Part model, mm, in its own coordinate system. Give positions to 0.01 mm unless a question says otherwise; leave off trailing zeros. Write each loop counter-clockwise with the first axis right and the second up, starting at its lowest first coordinate (ties: lowest second). Pieces come first, ordered by that corner, then holes. Notation, with made-up numbers: M -25.75,9.25 L 32.25,9.25 A34 ccw 32.25,39.25 Z; hole C 22,28.25 d4. An arc over 180 degrees is marked long. Use CSV: the item, a comma, the result in double quotes. Start each with the question number.
Item 1: Mould opens along Y. For faces 1 (the flat face through (-14, 704.486, 30)), 2 (the cylindrical face through (7.331, 691.927, 29.671)), 3 (the flat face through (14.873, 689, 30)) say: released by +Y, released by -Y, zero draft, split by the parting line, or undercut.
Item 2: Drill centre lines: line 1 (X direction, y = 692.5, z = 19); line 2 (X direction, y = 691, z = -9); line 3 (Z direction, x = -22, y = 693). Where is each one in solid material? Low to high. Write a range as [from, to].
Item 3: Cut at A-A (x = -9). List the corners of the cut face in (y, z).
Item 4: Cut at D-D (z = 54.5). List the corners of the cut face in (x, y), then the cut area to 3 significant figures.
Item 5: Cut at B-B (z = 17). List the corners of the cut face in (x, y), then the cut area to 3 significant figures.
Item 6: Cut at C-C (y = 691). List the corners of the cut face in (x, z), then the cut area to 3 significant figures.
from build123d import *

# Parameters (mm, degrees)
BOSS_EXTRUDE1_DEPTH = 90
SKETCH3_R           = 11
CUT_EXTRUDE1_DEPTH  = 92.815774412
M6_TAPPED_HOLE_D    = 5


with BuildPart() as part:
    # Sketch1 → Boss-Extrude1 (new body)
    with BuildSketch(Plane(origin=(0, 2.518676762, -14.699029015), x_dir=(1, 0, 0), z_dir=(0, 0, 1))):
        Polygon((-43.126560257, 671.967635092), (-14.126560257, 671.967635092), (14.873439743, 671.967635092), (14.873439743, 701.967635092), (-43.126560257, 701.967635092), align=None)
    extrude(amount=BOSS_EXTRUDE1_DEPTH)

    # Sketch3 → Cut-Extrude1 (cut, through all)
    with BuildSketch(Plane.XZ.offset(-674.486311854)):
        with Locations(Location((-14.126560257, 15.300970985, 0), (0, 0, 270))):
            Circle(SKETCH3_R)
    extrude(amount=-CUT_EXTRUDE1_DEPTH, mode=Mode.SUBTRACT)

    # M6 Tapped Hole (through all)
    with Locations(Plane(origin=(545.719230148, 1586.957920749, 85.300970985), x_dir=(-1, 0, 0), z_dir=(0, 0, 1))):
        with Locations((514.845790405, 897.471608895), (537.845790405, 897.471608895), (581.845790405, 897.471608895), (604.845790405, 897.471608895), (514.845790405, 1450.886073068), (514.845790405, 1412.886073068), (537.845790405, 1453.886073068), (537.845790405, 1409.886073068), (581.845790405, 1453.886073068), (581.845790405, 1409.886073068), (604.845790405, 1450.886073068), (604.845790405, 1412.886073068), (514.845790405, 1431.886073068), (537.845790405, 1431.886073068), (581.845790405, 1431.886073068), (604.845790405, 1431.886073068)):
            Hole(M6_TAPPED_HOLE_D / 2)


solid = part.part
Worked answers:
1,face 1,"released by +Y"
1,face 2,"undercut"
1,face 3,"zero draft"
2,line 1,"x = [-43.13, -24.49], [-3.77, 14.87]"
2,line 2,"x = [-43.13, -38.12], [-34.14, 5.88], [9.86, 14.87]"
2,line 3,"z = [-14.7, 7.62], [22.98, 75.3]"
3,outline,"M 674.49,-14.7 L 704.49,-14.7 L 704.49,5.57 L 674.49,5.57 Z; M 674.49,25.03 L 704.49,25.03 L 704.49,75.3 L 674.49,75.3 Z"
4,outline,"M -43.13,674.49 L 14.87,674.49 L 14.87,704.49 L -43.13,704.49 Z; hole C -36.13,689.49 d5; hole C 7.87,689.49 d5"
4,area,"1,700 mm^2"
5,outline,"M -43.13,674.49 L -24.99,674.49 L -24.99,704.49 L -43.13,704.49 Z; M -3.26,674.49 L 14.87,674.49 L 14.87,704.49 L -3.26,704.49 Z; hole C -36.13,689.49 d5; hole C 7.87,689.49 d5"
5,area,"1,050 mm^2"
6,outline,"M -43.13,-14.7 L -38.12,-14.7 L -38.12,75.3 L -43.13,75.3 Z; M -34.14,-14.7 L 5.88,-14.7 L 5.88,75.3 L -34.14,75.3 Z; M 9.86,-14.7 L 14.87,-14.7 L 14.87,75.3 L 9.86,75.3 Z; hole C -14.13,15.3 d22"
6,area,"4,120 mm^2"
